```python
from build123d import *

# Parameters (mm, degrees)
SKETCH1_W           = 332.74
SKETCH1_H           = 193.04
BOSS_EXTRUDE1_DEPTH = 50.8
SKETCH2_R           = 20.216216718
SKETCH2_R_2         = 6.132571036
SKETCH2_R_3         = 5.692545101
SKETCH2_R_4         = 5.992355172
BOSS_EXTRUDE2_DEPTH = 6.35


with BuildPart() as part:
    # Sketch1 → Boss-Extrude1 (new body)
    with BuildSketch(Plane(origin=(0, 0, 0), x_dir=(1, 0, 0), z_dir=(0, 1, 0))):
        with Locations((-166.37, -96.52)):
            Rectangle(SKETCH1_W, SKETCH1_H)
    extrude(amount=BOSS_EXTRUDE1_DEPTH)

    # Sketch2 → Boss-Extrude2 (add)
    with BuildSketch(Plane(origin=(0, 0, 0), x_dir=(0, 0, -1), z_dir=(1, 0, 0))):
        with Locations((-126.480916113, 25.513488319)):
            Circle(SKETCH2_R)
        with Locations(Location((-166.882757539, 25.513488319, 0), (0, 0, 180))):
            Circle(SKETCH2_R_2)
        with Locations(Location((-69.963733445, 21.427908849, 0), (0, 0, 180))):
            Circle(SKETCH2_R_3)
        with Locations(Location((-37.279097685, 21.427908849, 0), (0, 0, 180))):
            Circle(SKETCH2_R_4)
    extrude(amount=BOSS_EXTRUDE2_DEPTH)


solid = part.part
```
Read the model definition and answer for the solid it produces. Units are mm, in the model's axes. A direction names the side the tool comes from. Coordinates: 2 decimals unless noted, no trailing zeros. Loops run counter-clockwise (first coordinate to the right, second up) from the corner with the lowest first, then second, coordinate; pieces in that order, holes last. Notation, with made-up numbers: (25.5, 15.25) - (32.5, 15.25) arc R10 cw to (32.5, 33.25) - close; hole circle Ø9 at (68.5, 89.5). An arc over 180 degrees is marked (long way). Answer in a Markdown table with one row per item.
1. Which of the six approach directions +Z, -Z, +X, -X, +Y, -Y give full straight-line access (tool end or side, diameter ignored) to faces 1 (the face through (-169, 50.8, 95)), 2 (the face through (0, 25, 98))?
Conclusion:
| item | result |
|---|---|
| face 1 | +Z, -Z, +X, -X, +Y |
| face 2 | +X |
2. Determine the mould class of faces 3 (the face through (-169, 25, 0)), 4 (the face through (6.35, 25, 167)), 5 (the face through (3.13, 31.59, 107.2)), 6 (the face through (-169, 25, 193.04)) for opening direction Z: +Z half, -Z half, draft (parallel to the pull), parting line (faces both ways), or undercut.
Conclusion:
| item | result |
|---|---|
| face 3 | -Z half |
| face 4 | draft |
| face 5 | undercut |
| face 6 | +Z half |
3. Given pin 1 (1.5 mm diameter, centred on y = 38, z = 30, fed in from +X), flat-ended and moving along its own axis, determine where the tip first touches the part or whether it passes through.
Conclusion:
| item | result |
|---|---|
| pin 1 | stops at x = 0 |
4. A straight line is drawn through the part: line 1 (X direction, y = 40, z = 57.5). Find the intervals that lie inside material, in ascending order.
Conclusion:
| item | result |
|---|---|
| line 1 | x = -332.74 to 0 |
5. Find section A-A, the plane z = 97.5. Write down the section's boundary in (x, y).
Conclusion:
| item | result |
|---|---|
| outline | (-332.74, 0) - (0, 0) - (0, 50.8) - (-332.74, 50.8) - close |
6. Find section B-B, the plane y = 41.5. Write down the section's boundary in (x, z).
Conclusion:
| item | result |
|---|---|
| outline | (-332.74, 0) - (0, 0) - (0, 114.11) - (6.35, 114.11) - (6.35, 138.86) - (0, 138.86) - (0, 193.04) - (-332.74, 193.04) - close |
